CAD build for the part. Positions are in the model's coordinates, mm. A direction names the side the tool comes from. Round coordinates to 2 decimals unless told otherwise and drop trailing zeros. Write each loop counter-clockwise with the first axis right and the second up, starting at its lowest first coordinate (ties: lowest second). Pieces come first, ordered by that corner, then holes. Notation, with made-up numbers: (-36, -40) - (-12, -40) arc R24 cw to (-12, -16) - close; hole circle Ø10 at (-19, -38). An arc over 180 degrees is marked (long way). Use one line per item in the form item = value. Start each with the question number.
Item 1: Pin check, flat tips, straight feed: pin 1 (0.9 mm diameter, centred on x = -49, z = -156, fed in from +Y); pin 2 (0.9 mm diameter, centred on x = -48, z = -263, fed in from -Y); pin 3 (1 mm diameter, centred on x = -19, z = -43, fed in from +Y). Stop position of each tip, or through.
Item 2: Pull direction Z, two halves, no side cores. Call faces 4 (the flat face through (-1, 1, 340)), 5 (the flat face through (1, 50, -269)), 6 (the flat face through (-1, 47, -256)): +Z half, -Z half, draft (parallel to the pull), parting line (faces both ways), or undercut.
Item 3: Band-saw the part on C-C, the plane z = -125.5. List the corners of the cut face in (x, y), and give its area (3 significant figures).
Item 4: Band-saw the part on A-A, the plane x = -9. List the corners of the cut face in (y, z).
Item 5: Drill centre lines: L1, parallel to X at y = 48.2, z = 283; L2, parallel to Z at x = 40, y = 49; L3, parallel to X at y = 11.5, z = 85. Where is each one in solid material? Low to high.
Item 6: Tool access for faces 1 (the flat face through (47, 11, -4)), 2 (the flat face through (-50, -10, 5)), 3 (the flat face through (1, -2, 310)): list every direction of +Z, -Z, +X, -X, +Y, -Y with a clear straight run to the whole face (end or side of a thin tool).
Item 7: Band-saw the part on B-B, the plane z = -209.5. List the corners of the cut face in (x, y), and give its area (3 significant figures).
Autodesk Inventor part; units mm, degrees
ref_plane "YZ Plane" through (0, 0, 0) normal (1, 0, 0) x (0, 1, 0)
ref_plane "XZ Plane" through (0, 0, 0) normal (0, 1, 0) x (-1, 0, 0)
ref_plane "XY Plane" through (0, 0, 0) normal (0, 0, 1) x (1, 0, 0)
sketch "Sketch1" plane through (0, 0, 0) normal (0, 0, 1) x (1, 0, 0)
  line L0 (-50, 50) -> (50, 50)
  line L1 (50, 50) -> (50, -50)
  line L2 (50, -50) -> (-50, -50)
  line L3 (-50, -50) -> (-50, 50)
  line L4 (-50, 50) -> (50, -50) construction
  line L5 (50, 50) -> (-50, -50) construction
  line L6 (-47, 47) -> (47, 47)
  line L7 (47, 47) -> (47, -47)
  line L8 (47, -47) -> (-47, -47)
  line L9 (-47, -47) -> (-47, 47)
  line L10 (-47, 47) -> (47, -47) construction
  line L11 (47, 47) -> (-47, -47) construction
  point P0 (0, 0)
  dimension "d0" = 100
  dimension "d1" = 100
  dimension "d2" = 94
  dimension "d3" = 94
extrude "Extrusion1" add sketch "Sketch1" along normal mid plane 620
sketch "Sketch3" plane through (50, -50, 310) normal (1, 0, 0) x (0, 0, -1)
  line L0 (310, 50) -> (40, 50)
  line L1 (310, 50) -> (620, 50)
  line L2 (620, 50) -> (330, 50)
  line L3 (40, 50) -> (330, 50)
  line L4 (40, 55.5) -> (620, 55.5)
  line L5 (620, 55.5) -> (620, 44.5)
  line L6 (620, 44.5) -> (40, 44.5)
  line L7 (40, 44.5) -> (40, 55.5)
  line L8 (40, 55.5) -> (620, 44.5) construction
  line L9 (620, 55.5) -> (40, 44.5) construction
  dimension "d6" = 270
  dimension "d7" = 310
  dimension "d23" = 290
  dimension "d24" = 580
  dimension "d25" = 11
extrude "Extrusion2" cut sketch "Sketch3" against normal blind 620
sketch "Sketch4" plane through (-50, 50, 310) normal (0, 1, 0) x (1, 0, 0)
  line L0 (50, 310) -> (50, 230)
  line L1 (50, 310) -> (50, 510)
  line L2 (50, 510) -> (50, 370)
  line L3 (0, 230) -> (100, 230)
  line L4 (100, 230) -> (100, 510)
  line L5 (100, 510) -> (0, 510)
  line L6 (0, 510) -> (0, 230)
  line L7 (0, 230) -> (100, 510) construction
  line L8 (100, 230) -> (0, 510) construction
  dimension "d12" = 80
  dimension "d13" = 200
  dimension "d14" = 140
extrude "Extrusion3" cut sketch "Sketch4" against normal blind 3
sketch "Sketch7" plane through (0, 0, 310) normal (0, 0, 1) x (1, 0, 0)
  line L0 (-50, -50) -> (50, -50)
  line L1 (-50, 50) -> (50, 50)
  line L2 (50, 50) -> (50, -50)
  line L3 (50, -50) -> (-50, -50)
  line L4 (-50, -50) -> (-50, 50)
  line L5 (-50, 50) -> (50, -50) construction
  line L6 (50, 50) -> (-50, -50) construction
  point P0 (0, 0)
extrude "Extrusion4" add sketch "Sketch7" along normal blind 30
mirror "Mirror1" about plane through (0, 0, 0) normal (0, 0, 1) of "Extrusion4"
sketch "Sketch9" plane through (-50, -50, 340) normal (0, -1, 0) x (1, 0, 0)
  line L0 (100, -30) -> (0, -30)
  line L1 (0, -30) -> (0, -650)
  line L2 (0, -650) -> (100, -650)
  line L3 (100, -650) -> (100, -30)
  line L4 (100, -30) -> (0, -650) construction
  line L5 (0, -30) -> (100, -650) construction
  line L6 (0, -30) -> (100, -30)
  line L7 (100, -30) -> (100, -100)
  line L8 (100, -100) -> (0, -100)
  line L9 (0, -100) -> (0, -30)
  line L10 (0, -650) -> (100, -650)
  line L11 (100, -650) -> (100, -580)
  line L12 (100, -580) -> (0, -580)
  line L13 (0, -580) -> (0, -650)
  point P0 (50, -340)
  dimension "d26" = 100
  dimension "d27" = 620
  dimension "d28" = 100
  dimension "d29" = 70
  dimension "d30" = 100
  dimension "d31" = 70
extrude "Extrusion6" cut sketch "Sketch9" against normal blind 3 contours L3 L8 L1 L0 | L3 L2 L1 L12
sketch "Sketch10" plane through (-50, 50, 80) normal (0, 1, 0) x (1, 0, 0)
  line L0 (100, -160) -> (0, -160)
  line L1 (0, -230) -> (100, -230)
  line L2 (0, -230) -> (100, -160)
  line L3 (10, -203) -> (90, -203)
  line L4 (90, -203) -> (90, -187)
  line L5 (90, -187) -> (10, -187)
  line L6 (10, -187) -> (10, -203)
  line L7 (10, -203) -> (90, -187) construction
  line L8 (90, -203) -> (10, -187) construction
  circle A0 centre (10, -187) radius 2.5
  circle A1 centre (10, -203) radius 2.5
  circle A2 centre (90, -203) radius 2.5
  circle A3 centre (90, -187) radius 2.5
  line L9 (72.5, -222.5) -> (27.5, -222.5)
  line L10 (27.5, -222.5) -> (27.5, -167.5)
  line L11 (27.5, -167.5) -> (72.5, -167.5)
  line L12 (72.5, -167.5) -> (72.5, -222.5)
  line L13 (72.5, -222.5) -> (27.5, -167.5) construction
  line L14 (27.5, -222.5) -> (72.5, -167.5) construction
  point P0 (50, 80)
  point P1 (50, -195)
  dimension "d34" = 80
  dimension "d35" = 16
  dimension "d36" = 5
  dimension "d37" = 5
  dimension "d38" = 5
  dimension "d39" = 5
  dimension "d42" = 45
  dimension "d43" = 55
extrude "Extrusion7" cut sketch "Sketch10" against normal blind 3 contours L10 L3 L2 | L2 L3 L12 L9 L10 | L3 L10 L5 L2 | L2 L5 L12 L3 | L5 L10 L11 L12 L2 | L2 L12 L5 | A1 L6 L3 | L3 L6 A1 | A2 L4 L3 | L3 L4 A2 | A0 L6 L5 | L5 L6 A0 | A3 L4 L5 | L5 L4 A3
properties part number "GUIA_CUADRADA"
Determined:
q1.pin_1 = 47
q1.pin_2 = -47
q1.pin_3 = -47
q2.face_4 = +Z half
q2.face_5 = draft
q2.face_6 = undercut
q3.outline = (-50, -50) - (50, -50) - (50, -5.5) - (47, -5.5) - (47, -47) - (-47, -47) - (-47, -5.5) - (-50, -5.5) - close; (-50, 5.5) - (-47, 5.5) - (-47, 47) - (-50, 47) - close; (47, 5.5) - (50, 5.5) - (50, 47) - (47, 47) - close
q3.area = 798 mm²
q4.outline = (-50, -340) - (50, -340) - (50, -200) - (47, -200) - (47, -310) - (-50, -310) - close; (-50, -240) - (-47, -240) - (-47, 240) - (-50, 240) - close; (-50, 310) - (47, 310) - (47, 302.5) - (50, 302.5) - (50, 340) - (-50, 340) - close; (47, 80) - (50, 80) - (50, 247.5) - (47, 247.5) - close
q5.L1 = -50 to -42.5, -37.5 to -22.5, 22.5 to 37.5, 42.5 to 50
q5.L2 = -340 to -200, 80 to 264.5, 269.5 to 280.5, 285.5 to 340
q5.L3 = -50 to -47, 47 to 50
q6.face_1 = none
q6.face_2 = +Z, -Z, -X, +Y, -Y
q6.face_3 = -Y
q7.outline = (-50, -50) - (50, -50) - (50, -5.5) - (47, -5.5) - (47, -47) - (-47, -47) - (-47, -5.5) - (-50, -5.5) - close; (-50, 5.5) - (-47, 5.5) - (-47, 47) - (47, 47) - (47, 5.5) - (50, 5.5) - (50, 50) - (-50, 50) - close
q7.area = 1,100 mm²
